The figure shows three views and two pictorial views of one solid part (mm, origin at its lowest corner). Answer the questions. A direction names the side the tool comes from. Round coordinates to 2 decimals unless told otherwise and drop trailing zeros. Order: outer loops, then holes, each group sorted by start corner. A loop starts at its lowest first (then second) coordinate and runs counter-clockwise, first axis right, second up. Notation, with made-up numbers: (45.25, 19.25) -> (66.25, 19.25) arc R19 cw to (66.25, 41.25) -> close; hole circle Ø6 at (64.5, 61). An arc over 180 degrees is marked (long way). One line per item, written item: value. Start each with the question number.
1. Section B-B (y = 12) is taken. Give the vertices of the cut face in (x, z).
2. Section A-A (z = 88) is taken. Give the vertices of the cut face in (x, y) (1 decimal), then the cut area to 3 significant figures.
3. For the marked faces 1 and 2, determine the directions among +Z, -Z, +X, -X, +Y, -Y from which every point of the face is accessible in a straight line to the end or side of a thin tool.
4. Section C-C (x = 121) is taken. Give the vertices of the cut face in (y, z), then the cut area to 3 significant figures.
5. A flat-ended cylindrical pin translates along its axis: pin 1 Ø9 at (x, y) = (94.5, 95) entering from +Z. Find the tip coordinate at first contact, or state that the pin passes through.
6. The mould has two halves that part along X. Classify the marked faces 3, 4, 5 and 6: released by +X, released by -X, zero draft, split by the parting line, or undercut.
7. Section D-D (z = 26) is taken. Give the vertices of the cut face in (x, y).
8. Consider line 1 (Y direction, x = 86, z = 40); line 2 (X direction, y = 33, z = 43). Determine where each line is inside the solid, lowest interval first.
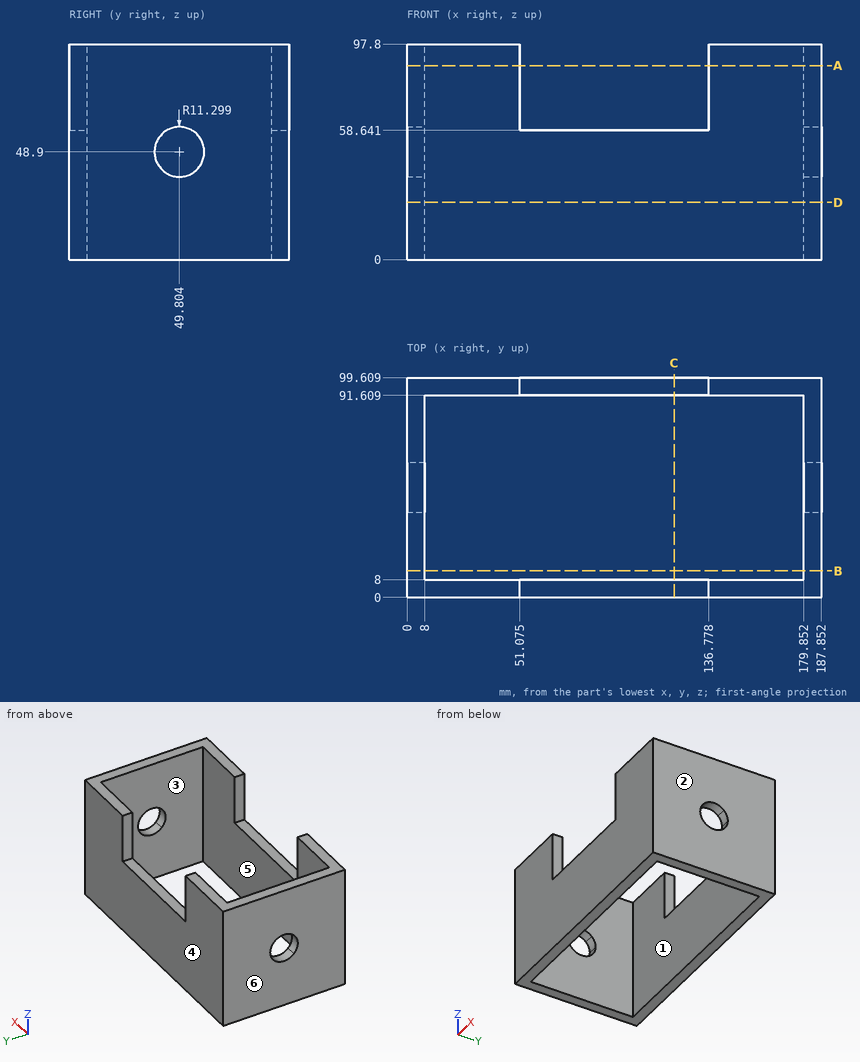
Answer:
1. outline: (0, 0) -> (8, 0) -> (8, 97.8) -> (0, 97.8) -> close; (179.85, 0) -> (187.85, 0) -> (187.85, 97.8) -> (179.85, 97.8) -> close
2. outline: (0, 0) -> (51.1, 0) -> (51.1, 8) -> (8, 8) -> (8, 91.6) -> (51.1, 91.6) -> (51.1, 99.6) -> (0, 99.6) -> close; (136.8, 0) -> (187.9, 0) -> (187.9, 99.6) -> (136.8, 99.6) -> (136.8, 91.6) -> (179.9, 91.6) -> (179.9, 8) -> (136.8, 8) -> close
2. area: 2,970 mm^2
3. face 1: +Z, -Z
3. face 2: +Z, -Z, +X, +Y, -Y
4. outline: (0, 0) -> (8, 0) -> (8, 58.64) -> (0, 58.64) -> close; (91.61, 0) -> (99.61, 0) -> (99.61, 58.64) -> (91.61, 58.64) -> close
4. area: 938 mm^2
5. pin 1: z = 58.64
6. face 3: undercut
6. face 4: zero draft
6. face 5: undercut
6. face 6: released by -X
7. outline: (0, 0) -> (187.85, 0) -> (187.85, 99.61) -> (0, 99.61) -> close; hole (8, 8) -> (179.85, 8) -> (179.85, 91.61) -> (8, 91.61) -> close
8. line 1: 0 to 8, 91.61 to 99.61
8. line 2: 0 to 8, 179.85 to 187.85
